Part model, mm, in its own coordinate system. Give positions to 0.01 mm unless a question says otherwise; leave off trailing zeros. Write each loop counter-clockwise with the first axis right and the second up, starting at its lowest first coordinate (ties: lowest second). Pieces come first, ordered by that corner, then holes.
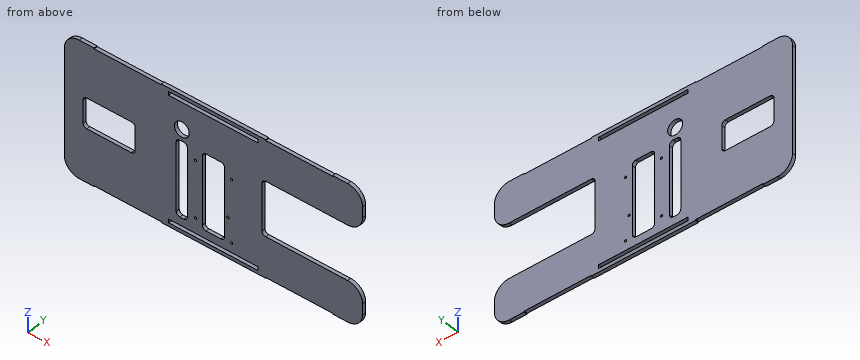
```python
from build123d import *

# Parameters (mm, degrees)
BOSS_EXTRUDE1_DEPTH = 2.38125
SKETCH2_W           = 135
SKETCH2_H           = 72
CUT_EXTRUDE1_DEPTH  = 10
SKETCH3_R           = 10
SKETCH3_W           = 15
SKETCH3_H           = 100
SKETCH3_W_2         = 70
SKETCH3_H_2         = 40
SKETCH3_W_3         = 30
CUT_EXTRUDE2_DEPTH  = 10
SKETCH4_R           = 1.5
CUT_EXTRUDE3_DEPTH  = 10
SKETCH5_W           = 120
SKETCH5_H           = 4.7625
CUT_EXTRUDE4_DEPTH  = 10
FILLET1_R           = 20
FILLET2_R           = 20
FILLET3_R           = 5


with BuildPart() as part:
    # Sketch1 → Boss-Extrude1 (new, symmetric)
    with BuildSketch(Plane(origin=(0, 0, 0), x_dir=(1, 0, 0), z_dir=(0, 1, 0))):
        Polygon((-200, 90), (-160, 90), (-160, 89), (-70, 89), (-70, 90), (70, 90), (70, 89), (160, 89), (160, 90), (200, 90), (200, -90), (160, -90), (160, -89), (70, -89), (70, -90), (-70, -90), (-70, -89), (-160, -89), (-160, -90), (-200, -90), align=None)
    extrude(amount=BOSS_EXTRUDE1_DEPTH, both=True)

    # Sketch2 → Cut-Extrude1 (cut)
    with BuildSketch(Plane(origin=(0, 2.38125, 0), x_dir=(1, 0, 0), z_dir=(0, 1, 0))):
        with Locations((132.5, 0)):
            Rectangle(SKETCH2_W, SKETCH2_H)
    extrude(amount=-CUT_EXTRUDE1_DEPTH, mode=Mode.SUBTRACT)

    # Sketch3 → Cut-Extrude2 (cut)
    with BuildSketch(Plane(origin=(0, 2.38125, 0), x_dir=(1, 0, 0), z_dir=(0, 1, 0))):
        with Locations(Location((-42.5, -45, 0), (0, 0, 270))):
            Circle(SKETCH3_R)
        with Locations((-42.5, 20)):
            Rectangle(SKETCH3_W, SKETCH3_H)
        with Locations((-140, 0)):
            Rectangle(SKETCH3_W_2, SKETCH3_H_2)
        with Locations((0, 20)):
            Rectangle(SKETCH3_W_3, SKETCH3_H)
    extrude(amount=-CUT_EXTRUDE2_DEPTH, mode=Mode.SUBTRACT)

    # Sketch4 → Cut-Extrude3 (cut)
    with BuildSketch(Plane(origin=(0, 2.38125, 0), x_dir=(1, 0, 0), z_dir=(0, 1, 0))):
        with Locations(Location((24.1681, -14.4776, 0), (0, 0, 270))):
            Circle(SKETCH4_R)
        with Locations(Location((-24.1681, -14.4776, 0), (0, 0, 270))):
            Circle(SKETCH4_R)
        with Locations(Location((-24.1681, 60.6556, 0), (0, 0, 270))):
            Circle(SKETCH4_R)
        with Locations(Location((24.1681, 68.1486, 0), (0, 0, 270))):
            Circle(SKETCH4_R)
        with Locations(Location((19.289607234, 37.1479, 0), (0, 0, 270))):
            Circle(SKETCH4_R)
    extrude(amount=-CUT_EXTRUDE3_DEPTH, mode=Mode.SUBTRACT)

    # Sketch5 → Cut-Extrude4 (cut)
    with BuildSketch(Plane(origin=(0, 2.38125, 0), x_dir=(1, 0, 0), z_dir=(0, 1, 0))):
        with Locations((0, 82.85625)):
            Rectangle(SKETCH5_W, SKETCH5_H)
        with Locations((0, -82.85625)):
            Rectangle(SKETCH5_W, SKETCH5_H)
    extrude(amount=-CUT_EXTRUDE4_DEPTH, mode=Mode.SUBTRACT)

    # Fillet1
    fillet1_edges = [part.edges().sort_by_distance(p)[0] for p in [
        (-200, 0, -90),
        (200, 0, -90),
        (200, 0, 90),
        (-200, 0, 90),
    ]]
    fillet(fillet1_edges, radius=FILLET1_R)

    # Fillet2
    fillet2_edges = [part.edges().sort_by_distance(p)[0] for p in [
        (200, 0, -36),
        (200, 0, 36),
    ]]
    fillet(fillet2_edges, radius=FILLET2_R)

    # Fillet3
    fillet3_edges = [part.edges().sort_by_distance(p)[0] for p in [
        (-175, 0, 20),
        (-175, 0, -20),
        (-105, 0, -20),
        (-105, 0, 20),
        (-35, 0, -70),
        (-35, 0, 30),
        (-50, 0, 30),
        (-50, 0, -70),
        (65, 0, 36),
        (65, 0, -36),
        (-15, 0, 30),
        (-15, 0, -70),
        (15, 0, -70),
        (15, 0, 30),
    ]]
    fillet(fillet3_edges, radius=FILLET3_R)


solid = part.part
```
1) Saw through at B-B, the plane z = -4.5. Write the cut outline in (x, y), then the cut area to 3 significant figures.
Answers follow:
outline: (-200, -2.38) - (-175, -2.38) - (-175, 2.38) - (-200, 2.38) - close; (-105, -2.38) - (-50, -2.38) - (-50, 2.38) - (-105, 2.38) - close; (-35, -2.38) - (-15, -2.38) - (-15, 2.38) - (-35, 2.38) - close; (15, -2.38) - (65, -2.38) - (65, 2.38) - (15, 2.38) - close
area: 714 mm2
2) Wall check: L1, parallel to Z at x = 19, y = 0.2 (1 decimal); L2, parallel to X at y = 0.6, z = -6; L3, parallel to X at y = 0.8, z = -21. Give the ranges that are in metal, low to high.
Answers follow:
L1: z = -90 to -85.2, -80.5 to -38.6, -35.7 to 80.5, 85.2 to 90
L2: x = -200 to -175, -105 to -50, -35 to -15, 15 to 65
L3: x = -200 to -50, -35 to -15, 15 to 65
3) Saw through at D-D, the plane z = -48. Write the cut outline in (x, y), then the cut area to 3 significant figures.
Answers follow:
outline: (-200, -2.38) - (-50, -2.38) - (-50, 2.38) - (-200, 2.38) - close; (-35, -2.38) - (-15, -2.38) - (-15, 2.38) - (-35, 2.38) - close; (15, -2.38) - (198.33, -2.38) - (198.33, 2.38) - (15, 2.38) - close
area: 1,680 mm2
4) Pin check, flat tips, straight feed: pin 1 Ø1.5 at (x, y) = (119, 1.5) entering from +Z; pin 2 Ø2.5 at (x, y) = (144.5, 0) entering from -Z; pin 3 Ø1.4 at (y, z) = (0, -22) entering from +X. Stop position of each tip, or through.
Answers follow:
pin 1: stops at z = 89
pin 2: stops at z = -89
pin 3: stops at x = 65
5) Saw through at C-C, the plane x = 50.5. Write the cut outline in (y, z) (1 decimal), then the cut area to 3 significant figures.
Answers follow:
outline: (-2.4, -90) - (2.4, -90) - (2.4, -85.2) - (-2.4, -85.2) - close; (-2.4, -80.5) - (2.4, -80.5) - (2.4, 80.5) - (-2.4, 80.5) - close; (-2.4, 85.2) - (2.4, 85.2) - (2.4, 90) - (-2.4, 90) - close
area: 812 mm2
6) Saw through at A-A, the plane x = -165. Write the cut outline in (y, z), then the cut area to 3 significant figures.
Answers follow:
outline: (-2.38, -90) - (2.38, -90) - (2.38, -20) - (-2.38, -20) - close; (-2.38, 20) - (2.38, 20) - (2.38, 90) - (-2.38, 90) - close
area: 667 mm2
